Read the model definition and answer for the solid it produces. Units are mm, in the model's axes. Round coordinates to 2 decimals unless told otherwise and drop trailing zeros. Loops run counter-clockwise (first coordinate to the right, second up) from the corner with the lowest first, then second, coordinate; pieces in that order, holes last. Notation, with made-up numbers: (-19.5, -35) - (5.5, -35) arc R20 cw to (5.5, -30) - close; hole circle Ø8 at (-23, 6.5). An arc over 180 degrees is marked (long way). Use one line per item in the form item = value. Start each with the question number.
```python
from build123d import *

# Parameters (mm, degrees)
SKETCH1_R           = 41
SKETCH1_R_2         = 39
BOSS_EXTRUDE1_DEPTH = 10
SKETCH2_R           = 41
SKETCH2_R_2         = 36
BOSS_EXTRUDE2_DEPTH = 2
BOSS_EXTRUDE3_START = 2
SKETCH3_R           = 41
SKETCH3_R_2         = 36.3
BOSS_EXTRUDE3_DEPTH = 2
FILLET2_R           = 5
FILLET6_R           = 7


with BuildPart() as part:
    # Sketch1 → Boss-Extrude1 (new body)
    with BuildSketch(Plane.XY):
        Circle(SKETCH1_R)
        Circle(SKETCH1_R_2, mode=Mode.SUBTRACT)
    extrude(amount=BOSS_EXTRUDE1_DEPTH)

    # Sketch2 → Boss-Extrude2 (add)
    with BuildSketch(Plane.XY.offset(10)):
        Circle(SKETCH2_R)
        Circle(SKETCH2_R_2, mode=Mode.SUBTRACT)
    extrude(amount=BOSS_EXTRUDE2_DEPTH)

    # Sketch3 → Boss-Extrude3 (add)
    with BuildSketch(Plane(origin=(0, 0, 0), x_dir=(-1, 0, 0), z_dir=(0, 0, -1)).offset(BOSS_EXTRUDE3_START)):
        Circle(SKETCH3_R)
        Circle(SKETCH3_R_2, mode=Mode.SUBTRACT)
    extrude(amount=-BOSS_EXTRUDE3_DEPTH)

    # Fillet2
    # the kernel refuses this fillet: 5 mm, written as the material it adds along each edge
    with BuildSketch(Plane(origin=(0, 0, 10), x_dir=(1, 0, 0), z_dir=(0, -1, 0))) as fillet2_piece_1:
        with BuildLine():
            CenterArc((34, -4.582575695), FILLET2_R, 0, 66.421821522)
            Line((39, -4.582575695), (39.1, -4.582575695))
            Line((39.1, -4.582575695), (39.1, 0))
            Line((39.1, 0), (39, 0.1))
            ThreePointArc((39, 0.1), (37.5, 0.1), (36.04, 0.091651514))
            Line((36.04, 0.091651514), (36, 0))
        make_face()
    revolve(axis=Axis((0, 0, 10), (0, 0, 1)))
    with BuildSketch(Plane(origin=(0, 0, 0), x_dir=(1, 0, 0), z_dir=(0, -1, 0))) as fillet2_piece_2:
        with BuildLine():
            CenterArc((34, 4.439594576), FILLET2_R, 297.387107503, 62.612892497)
            Line((36.3, 0), (36.346, -0.088791892))
            ThreePointArc((36.346, -0.088791892), (37.65, -0.1), (39, -0.1))
            Line((39, -0.1), (39.1, 0))
            Line((39.1, 0), (39.1, 4.439594576))
            Line((39.1, 4.439594576), (39, 4.439594576))
        make_face()
    revolve(axis=Axis((0, 0, 0), (0, 0, 1)))

    # Fillet6
    # the kernel refuses this fillet: 7 mm, written as the material it takes off along each edge
    with BuildSketch(Plane(origin=(0, 0, -2), x_dir=(-1, 0, 0), z_dir=(0, -1, 0))) as fillet6_piece_1:
        with BuildLine():
            CenterArc((34, -6.61135387), FILLET6_R, 0, 70.817910057)
            Line((41, -6.61135387), (41.14, -6.61135387))
            Line((41.14, -6.61135387), (41.14, 0))
            Line((41.14, 0), (41, 0.14))
            ThreePointArc((41, 0.14), (38.65, 0.14), (36.346, 0.132227077))
            Line((36.346, 0.132227077), (36.3, 0))
        make_face()
    revolve(axis=Axis((0, 0, -2), (0, 0, -1)), mode=Mode.SUBTRACT)
    with BuildSketch(Plane(origin=(0, 0, 12), x_dir=(1, 0, 0), z_dir=(0, -1, 0))) as fillet6_piece_2:
        with BuildLine():
            CenterArc((34, -6.708203932), FILLET6_R, 0, 73.398450401)
            Line((36, 0), (36.04, 0.134164079))
            ThreePointArc((36.04, 0.134164079), (38.5, 0.14), (41, 0.14))
            Line((41, 0.14), (41.14, 0))
            Line((41.14, 0), (41.14, -6.708203932))
            Line((41.14, -6.708203932), (41, -6.708203932))
        make_face()
    revolve(axis=Axis((0, 0, 12), (0, 0, 1)), mode=Mode.SUBTRACT)


solid = part.part
```
1) Determine the mould class of faces 1 (the cylindrical face through (-5.077, 38.668, 4.922)), 2 (the cylindrical face through (18.919, 36.374, 4.947)), 3 (the cylindrical face through (-4.686, 35.694, 10.986)) for opening direction X: +X half, -X half, draft (parallel to the pull), parting line (faces both ways), or undercut.
2) Flat-ended cylindrical pins translate along their axes: pin 1 (4 mm diameter, centred on y = -31, z = 0, fed in from -X); pin 2 (4 mm diameter, centred on x = -29.5, z = 5.5, fed in from -Y); pin 3 (1.5 mm diameter, centred on x = -16, z = 2, fed in from +Y). Find the tip coordinate at first contact, or state that the pin passes through.
3) A cutting plane is placed at D-D on z = 8.75. Write down the section's boundary in (x, y).
4) A cutting plane is placed at C-C on z = 1. Write down the section's boundary in (x, y), plus the area to 3 significant figures.
5) A cutting plane is placed at A-A on x = 0. Write down the section's boundary in (y, z), plus the area to 3 significant figures.
6) Straight lines are drawn through the part: line 1 (Y direction, x = -22, z = 6.75); line 2 (X direction, y = 35, z = 6.25); line 3 (X direction, y = -15, z = 3). For each, find the intervals that lie inside material, in ascending order. Write a range as from..to.
Checks:
q1.face_1 = undercut
q1.face_2 = parting line
q1.face_3 = undercut
q2.pin_1 = -27.29
q2.pin_2 = -30.41
q2.pin_3 = 37.63
q3.outline = circle Ø80.17 at (0, 0); hole circle Ø75.45 at (0, 0)
q4.outline = circle Ø79.99 at (0, 0); hole circle Ø75.26 at (0, 0)
q4.area = 577 mm²
q5.outline = (-41, 4.61) arc R7 ccw to (-36.3, -2) - (-36.3, 0) arc R5 cw to (-39, 4.44) - (-39, 5.42) arc R5 cw to (-36, 10) - (-36, 12) arc R7 ccw to (-41, 5.29) - close; (36, 10) arc R5 cw to (39, 5.42) - (39, 4.44) arc R5 cw to (36.3, 0) - (36.3, -2) arc R7 ccw to (41, 4.61) - (41, 5.29) arc R7 ccw to (36, 12) - close
q5.area = 58.8 mm²
q6.line_1 = -34.42..-31.98, 31.98..34.42
q6.line_2 = -21.23..-17.05, 17.05..21.23
q6.line_3 = -37.96..-35.77, 35.77..37.96
